Check sheet for the modelled part. Datum: model origin and axes. Units: mm. Face numbers are marked on the shaded views. A direction names the side the tool comes from. Give positions to 0.01 mm unless a question says otherwise; leave off trailing zeros. Write each loop counter-clockwise with the first axis right and the second up, starting at its lowest first coordinate (ties: lowest second). Pieces come first, ordered by that corner, then holes. Notation, with made-up numbers: M 39,-24 L 89,-24 A30 cw 89,5 Z; hole C 23.25,-24 d1. An arc over 180 degrees is marked long. Use CSV: the item, a comma, the result in double quotes. Start each with the question number.
1. Mould release check, pull along Y, two halves, no side actions. Record for the marked faces 3, 4, 5 and 6: +Y half, -Y half, draft (parallel to the pull), parting line (faces both ways), or undercut.
2. Cross-section at D-D, the plane x = -7. Enter the section's corners in (y, z).
3. Scan lines: line 1 (Y direction, x = 0, z = 1.6); line 2 (Z direction, x = 17.5, y = -14); line 3 (Y direction, x = 0.5, z = 4.25). Record each from-to range of solid material in increasing order.
4. Cross-section at A-A, the plane z = 2.25. Enter the section's corners in (x, y), and give its area (3 significant figures).
5. Access from +Z, -Z, +X, -X, +Y, -Y to the whole of each face (thin tool, end or side, straight path). Record for the marked faces 1 and 2.
6. Depth check by flat-ended pin: P1, Ø1, axis at x = 6, z = 8.5, coming from the -Y side; P2, Ø6, axis at x = -4, y = 4, coming from the +Z side; P3, Ø0.9, axis at y = 1.5, z = 8.5, coming from the +X side. Enter the tip coordinate at first touch or a pass-through.
7. Cross-section at C-C, the plane y = -18. Enter the section's corners in (x, z), and give its area (3 significant figures).
8. Cross-section at B-B, the plane z = 8. Enter the section's corners in (x, y).
from build123d import *

# Parameters (mm, degrees)
BOX_W             = 20
BOX_H             = 20
BOX_DEPTH         = 20
CIRCLE001_R       = 19
EXTRUDE001_DEPTH  = 10
CYLINDER001_R     = 0.5
CYLINDER001_DEPTH = 10
CYLINDER002_R     = 0.5
CYLINDER002_DEPTH = 10
CYLINDER003_R     = 0.5
CYLINDER003_DEPTH = 10
CYLINDER_R        = 0.5
CYLINDER_DEPTH    = 10
CIRCLE_R          = 24
EXTRUDE_DEPTH     = 4


with BuildPart() as cube:
    # Box → Box (new body)
    with BuildSketch(Plane(origin=(-10, -10, 7), x_dir=(1, 0, 0), z_dir=(0, 0, 1))):
        with Locations((10, 10)):
            Rectangle(BOX_W, BOX_H)
    extrude(amount=BOX_DEPTH)


with BuildPart() as extrude001:
    # Circle001 → Extrude001 (new body)
    with BuildSketch(Plane.XY):
        Circle(CIRCLE001_R)
    extrude(amount=EXTRUDE001_DEPTH)


with BuildPart() as cylinder001:
    # Cylinder001 → Cylinder001 (new body)
    with BuildSketch(Plane(origin=(-21.5, 0, -3), x_dir=(1, 0, 0), z_dir=(0, 0, 1))):
        Circle(CYLINDER001_R)
    extrude(amount=CYLINDER001_DEPTH)


with BuildPart() as cylinder002:
    # Cylinder002 → Cylinder002 (new body)
    with BuildSketch(Plane(origin=(0, 21.5, -3), x_dir=(1, 0, 0), z_dir=(0, 0, 1))):
        Circle(CYLINDER002_R)
    extrude(amount=CYLINDER002_DEPTH)


with BuildPart() as cylinder003:
    # Cylinder003 → Cylinder003 (new body)
    with BuildSketch(Plane(origin=(0, -21.5, -3), x_dir=(1, 0, 0), z_dir=(0, 0, 1))):
        Circle(CYLINDER003_R)
    extrude(amount=CYLINDER003_DEPTH)


with BuildPart() as fusion:
    # Cylinder → Cylinder (new body)
    with BuildSketch(Plane(origin=(21.5, 0, -3), x_dir=(1, 0, 0), z_dir=(0, 0, 1))):
        Circle(CYLINDER_R)
    extrude(amount=CYLINDER_DEPTH)

    # Fusion: union Cylinder001, Cylinder002, Cylinder003
    add(cylinder001.part)
    add(cylinder002.part)
    add(cylinder003.part)


with BuildPart() as cut001:
    # Circle → Extrude (new body)
    with BuildSketch(Plane.XY):
        Circle(CIRCLE_R)
    extrude(amount=EXTRUDE_DEPTH)

    # Cut: cut Fusion
    add(fusion.part, mode=Mode.SUBTRACT)

    # Fusion001: union Extrude001
    add(extrude001.part)

    # Cut001: cut Cube
    add(cube.part, mode=Mode.SUBTRACT)


solid = cut001.part
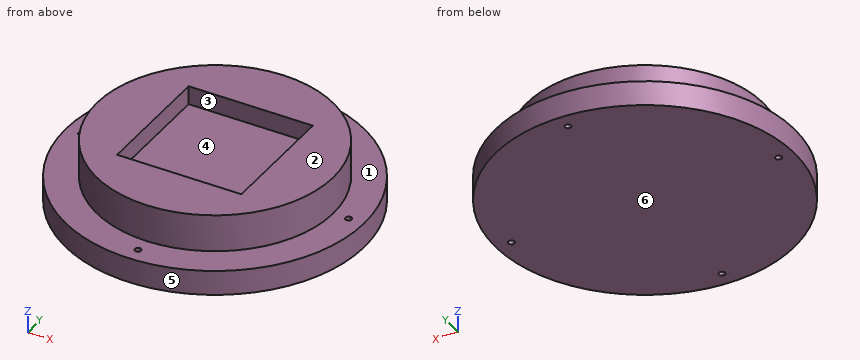
Worked answers:
1,face 3,"undercut"
1,face 4,"undercut"
1,face 5,"parting line"
1,face 6,"draft"
2,outline,"M -22.96,0 L 22.96,0 L 22.96,4 L 17.66,4 L 17.66,10 L 10,10 L 10,7 L -10,7 L -10,10 L -17.66,10 L -17.66,4 L -22.96,4 Z"
3,line 1,"y = -24 to -22, -21 to 21, 22 to 24"
3,line 2,"z = 0 to 4"
3,line 3,"y = -18.99 to 18.99"
4,outline,"C 0,0 d48; hole C -21.5,0 d1; hole C 0,-21.5 d1; hole C 0,21.5 d1; hole C 21.5,0 d1"
4,area,"1,810 mm^2"
5,face 1,"+Z"
5,face 2,"+Z, +X, -X, +Y, -Y"
6,P1,"stops at y = -18.19"
6,P2,"stops at z = 7"
6,P3,"stops at x = 18.97"
7,outline,"M -15.87,0 L 15.87,0 L 15.87,4 L 6.08,4 L 6.08,10 L -6.08,10 L -6.08,4 L -15.87,4 Z"
7,area,"200 mm^2"
8,outline,"C 0,0 d38; hole M -10,-10 L 10,-10 L 10,10 L -10,10 Z"
